Autodesk Inventor part; units mm, degrees
ref_plane "YZ Plane" through (0, 0, 0) normal (1, 0, 0) x (0, 1, 0)
ref_plane "XZ Plane" through (0, 0, 0) normal (0, 1, 0) x (-1, 0, 0)
ref_plane "XY Plane" through (0, 0, 0) normal (0, 0, 1) x (1, 0, 0)
sketch "Schizzo1" plane through (0, 0, 0) normal (0, 1, 0) x (-1, 0, 0)
  line L0 (25, 50) -> (-25, 50)
  line L1 (-25, 50) -> (-25, -50)
  line L2 (-25, -50) -> (25, -50)
  line L3 (25, -50) -> (25, 50)
  line L4 (25, 50) -> (-25, -50) construction
  line L5 (-25, 50) -> (25, -50) construction
  point P0 (0, 0)
  point P1 (0, 0)
  point P2 (0, 0)
  dimension "d0" = 50
  dimension "d9" = 100
extrude "Estrusione1" add sketch "Schizzo1" along normal blind 16
sketch "Schizzo2" plane through (0, 0, 0) normal (0, -1, 0) x (1, 0, 0)
  circle A0 centre (25, 0) radius 9.5
  line L0 (25, 50) -> (25, -50)
  point P0 (0, 0)
  dimension "d3" = 19
extrude "Estrusione2" cut sketch "Schizzo2" against normal blind 4
sketch "Schizzo4" plane through (0, 4, 0) normal (0, -1, 0) x (1, 0, 0)
  circle A0 centre (25, 0) radius 6
  line L0 (25, 9.5) -> (25, -9.5)
  point P0 (0, 0)
  point P1 (25, 6)
  point P2 (25, -6)
  dimension "d6" = 12
extrude "Estrusione3" cut sketch "Schizzo4" against normal blind 26 contours L0 A0 picked at (23.13, -0.7092)
sketch "Schizzo5" plane through (-25, 0, -50) normal (-1, 0, 0) x (0, 0, 1)
  line L0 (50, 0) -> (50, 8)
  line L1 (50, 8) -> (75, 8)
  line L2 (50, 8) -> (25, 8)
  line L3 (50, 8) -> (75, 8) construction
  dimension "d10" = 8
  dimension "d11" = 25
  dimension "d12" = 25
  dimension "d13" = 180
hole "Foro1" at (-25, 8, -25) at (-25, 8, 25) direction (1, 0, 0) diameter 6.6 end through all
sketch "Schizzo6" plane through (-25, 0, -50) normal (-1, 0, 0) x (0, 0, 1)
  circle A0 centre (25, 8) radius 3.3
  circle A1 centre (25, 8) radius 5
  circle A2 centre (75, 8) radius 3.3
  circle A3 centre (75, 8) radius 5
  circle A4 centre (25, 8) radius 3.3
  line L0 (27.8868, 13) -> (30.7735, 8)
  line L1 (30.7735, 8) -> (27.8868, 3)
  line L2 (27.8868, 3) -> (22.1132, 3)
  line L3 (22.1132, 3) -> (19.2265, 8)
  line L4 (19.2265, 8) -> (22.1132, 13)
  line L5 (22.1132, 13) -> (27.8868, 13)
  line L6 (77.8868, 13) -> (80.7735, 8)
  line L7 (80.7735, 8) -> (77.8868, 3)
  line L8 (77.8868, 3) -> (72.1132, 3)
  line L9 (72.1132, 3) -> (69.2265, 8)
  line L10 (69.2265, 8) -> (72.1132, 13)
  line L11 (72.1132, 13) -> (77.8868, 13)
  point P0 (50, 0)
  point P1 (25, 13)
  point P2 (75, 13)
  dimension "d21" = 10
  dimension "d22" = 10
extrude "Estrusione4" cut sketch "Schizzo6" against normal blind 6 contours A0 | A1 | A1 L0 L1 | A1 L5 L0 | L1 L2 A1 | A1 L4 L5 | L2 L3 A1 | A1 L3 L4 | A2 | A3 | A3 L6 L7 | A3 L11 L6 | L7 L8 A3 | A3 L10 L11 | L8 L9 A3 | A3 L9 L10
properties part number "15_Base_Dietro"
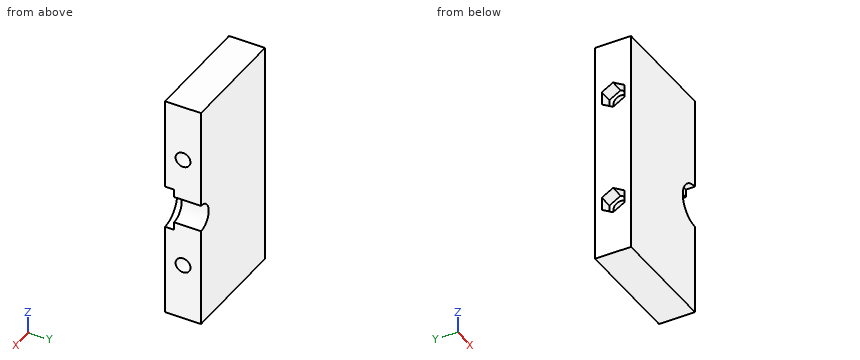
CAD build for the part. Positions are in the model's coordinates, mm. Round coordinates to 2 decimals unless told otherwise and drop trailing zeros. Loops run counter-clockwise (first coordinate to the right, second up) from the corner with the lowest first, then second, coordinate; pieces in that order, holes last. Notation, with made-up numbers: M 34.5,7 L 58.5,7 A18 ccw 58.5,26 Z; hole C 23.25,47.25 d6. An arc over 180 degrees is marked long. One line per question, with ' | ' between items. Start each with the question number.
Item 1: Cut at D-D, the plane z = 0. Write the cut outline in (x, y), plus the area to 3 significant figures.
Item 2: Wall check: line 1 (Z direction, x = 4, y = 8); line 2 (Y direction, x = 6, z = 25); line 3 (Z direction, x = -4.5, y = 5.25). Give the ranges that are in metal, low to high.
Item 3: Cut at B-B, the plane y = 9. Write the cut outline in (x, z).
Item 4: Cut at A-A, the plane z = -25. Write the cut outline in (x, y).
Item 5: Cut at C-C, the plane x = -16.5. Write the cut outline in (y, z), plus the area to 3 significant figures.
Item 6: Pin check, flat tip, straight feed: pin 1 Ø7.5 at (y, z) = (8, 25) entering from -X. Stop position of the tip, or through.
Responses:
1) outline: M -25,0 L 15.5,0 L 15.5,4 L 19,4 L 19,16 L -25,16 Z | area: 690 mm²
2) line 1: z = -50 to -28.3, -21.7 to 21.7, 28.3 to 50 | line 2: y = 0 to 4.7, 11.3 to 16 | line 3: z = -50 to -26.82, -23.18 to 23.18, 26.82 to 50
3) outline: M -25,-50 L 25,-50 L 25,-28.14 L -19,-28.14 L -19,-30.2 L -25,-30.2 Z; M -25,-19.8 L -19,-19.8 L -19,-21.86 L 25,-21.86 L 25,-6 A6 cw 25,6 L 25,21.86 L -19,21.86 L -19,19.8 L -25,19.8 Z; M -25,30.2 L -19,30.2 L -19,28.14 L 25,28.14 L 25,50 L -25,50 Z
4) outline: M -25,0 L 25,0 L 25,4.7 L -19,4.7 L -19,3 L -25,3 Z; M -25,13 L -19,13 L -19,11.3 L 25,11.3 L 25,16 L -25,16 Z
5) outline: M 0,-50 L 16,-50 L 16,50 L 0,50 Z; hole C 8,-25 d6.6; hole C 8,25 d6.6 | area: 1,530 mm²
6) pin 1: stops at x = -19
